from build123d import *

# Parameters (mm, degrees)
F0_R     = 2.3
F1_DEPTH = 19
F3_DEPTH = 43.4
F5_R     = 6.25
F6_DEPTH = 20
F7_R     = 5.375
F8_DEPTH = 12


with BuildPart() as f1:
    # F0 (on Top) → F1 (new body)
    with BuildSketch(Plane.XY):
        with BuildLine():
            Line((84.03, 17.5), (-7.5, 17.5))
            ThreePointArc((-7.5, 17.5), (-12.908327, 15.86249), (-16.5, 11.5))
            Line((-16.5, 11.5), (-16.5, -11.5))
            ThreePointArc((-16.5, -11.5), (-12.908327, -15.86249), (-7.5, -17.5))
            Line((-7.5, -17.5), (84.03, -17.5))
            ThreePointArc((84.03, -17.5), (89.438327, -15.86249), (93.03, -11.5))
            Line((93.03, -11.5), (93.03, 11.5))
            ThreePointArc((93.03, 11.5), (89.438327, 15.86249), (84.03, 17.5))
        make_face()
        Circle(F0_R, mode=Mode.SUBTRACT)
        with Locations((70.419462, 0)):
            Circle(F0_R, mode=Mode.SUBTRACT)
    extrude(amount=F1_DEPTH)

    # F2 (on face) → F3 (join)
    with BuildSketch(Plane.XY.offset(19)):
        Polygon((14.9, 17.5), (14.9, 0), (14.9, -17.5), (51.9, -17.5), (51.9, 0), (51.9, 17.5), align=None)
    extrude(amount=F3_DEPTH)

    # F5 (on face) → F6 (cut)
    with BuildSketch(Plane.YZ.offset(51.9)):
        with Locations((0, 48)):
            Circle(F5_R)
    extrude(amount=-F6_DEPTH, mode=Mode.SUBTRACT)

    # F7 (on face) → F8 (cut)
    with BuildSketch(Plane.XY.offset(19)):
        Circle(F7_R)
        with Locations((70.419462, 0)):
            Circle(F7_R)
    extrude(amount=-F8_DEPTH, mode=Mode.SUBTRACT)


solid = f1.part
Design review of the part built by this model. Coordinates are the model's own, in mm. A direction names the side the tool comes from. Round coordinates to 2 decimals unless told otherwise and drop trailing zeros. Loops run counter-clockwise (first coordinate to the right, second up) from the corner with the lowest first, then second, coordinate; pieces in that order, holes last. Notation, with made-up numbers: (-25.5, 40.25) -> (24.5, 40.25) arc R22 ccw to (24.5, 69.25) -> close; hole circle Ø1 at (25.25, 30.5). An arc over 180 degrees is marked (long way). Use one line per item in the form item = value. Start each with the question number.
Q1. We need section B-B on y = 0. Give the boundary of the cut face in (x, z) (3 decimals).
Q2. Machinability: for faces 5 (the face through (-12.84, 15.91, 9.37)), 6 (the face through (1.1, -2.3, 7)), 7 (the face through (42, -0.8, 54.2)), 8 (the face through (77, 0, 19)), 9 (the face through (14.9, 0, 40)), which of the approach directions +Z, -Z, +X, -X, +Y, -Y give a long, thin tool a straight path to every point of the face, cutting with its end or side? Answer none if there is none.
Q3. We need section D-D on y = 10. Give the boundary of the cut face in (x, z), then the cut area to 3 significant figures.
Q4. Draft analysis for pull direction X (two halves, no side actions). For faces 1 (the face through (51.9, 0, 40)), 2 (the face through (33, 0, 62.4)), 3 (the face through (-13, -15.8, 9.4)), 4 (the face through (68.12, 0.1, 3.45)), state which applies: +X half, -X half, draft (parallel to the pull), parting line (faces both ways), or undercut.
Q5. We need section A-A on x = 0. Give the boundary of the cut face in (y, z) (3 decimals), then the cut area to 3 significant figures.
Q6. Wall thickness on line 1 along X through (y, z) = (0, 5); line 2 along Z through (x, y) = (36, 0); line 3 along X through (y, z) = (6, 42): over which ranges is each line inside the solid? List them lowest first. Write a range as [from, to].
Q7. We need section C-C on z = 15. Give the boundary of the cut face in (x, y) (3 decimals), then the cut area to 3 significant figures.
Q8. For pin 1 Ø14.5 at (y, z) = (0, 48) entering from -X; pin 2 Ø5.5 at (x, y) = (0, 0) entering from +Z; pin 3 Ø10.5 at (y, z) = (6.5, 42) entering from +X, all flat-tipped, find the tip position at first contact; note any pin that passes through.
Calculated:
q1.outline = (-16.5, 0) -> (-2.3, 0) -> (-2.3, 7) -> (-5.375, 7) -> (-5.375, 19) -> (-16.5, 19) -> close; (2.3, 0) -> (68.119, 0) -> (68.119, 7) -> (65.044, 7) -> (65.044, 19) -> (51.9, 19) -> (51.9, 41.75) -> (31.9, 41.75) -> (31.9, 54.25) -> (51.9, 54.25) -> (51.9, 62.4) -> (14.9, 62.4) -> (14.9, 19) -> (5.375, 19) -> (5.375, 7) -> (2.3, 7) -> close; (72.719, 0) -> (93.03, 0) -> (93.03, 19) -> (75.794, 19) -> (75.794, 7) -> (72.719, 7) -> close
q2.face_5 = +Z, -Z, -X, +Y
q2.face_6 = +Z
q2.face_7 = +X
q2.face_8 = +Z, +X, +Y, -Y
q2.face_9 = +Z, -X, +Y, -Y
q3.outline = (-16.5, 0) -> (93.03, 0) -> (93.03, 19) -> (51.9, 19) -> (51.9, 62.4) -> (14.9, 62.4) -> (14.9, 19) -> (-16.5, 19) -> close
q3.area = 3,690 mm²
q4.face_1 = +X half
q4.face_2 = draft
q4.face_3 = -X half
q4.face_4 = undercut
q5.outline = (-17.5, 0) -> (-2.3, 0) -> (-2.3, 7) -> (-5.375, 7) -> (-5.375, 19) -> (-17.5, 19) -> close; (2.3, 0) -> (17.5, 0) -> (17.5, 19) -> (5.375, 19) -> (5.375, 7) -> (2.3, 7) -> close
q5.area = 504 mm²
q6.line_1 = [-16.5, -2.3], [2.3, 68.12], [72.72, 93.03]
q6.line_2 = [0, 41.75], [54.25, 62.4]
q6.line_3 = [14.9, 51.9]
q7.outline = (-16.5, -11.5) arc R9.75 ccw to (-7.5, -17.5) -> (84.03, -17.5) arc R9.75 ccw to (93.03, -11.5) -> (93.03, 11.5) arc R9.75 ccw to (84.03, 17.5) -> (-7.5, 17.5) arc R9.75 ccw to (-16.5, 11.5) -> close; hole circle Ø10.75 at (0, 0); hole circle Ø10.75 at (70.419, 0)
q7.area = 3,590 mm²
q8.pin_1 = 14.9
q8.pin_2 = 7
q8.pin_3 = 51.9
